For this review, take the finished solid that the model builds, in its own axes (mm). A direction names the side the tool comes from. Round coordinates to 2 decimals unless told otherwise and drop trailing zeros. Order: outer loops, then holes, each group sorted by start corner. A loop starts at its lowest first (then second) coordinate and runs counter-clockwise, first axis right, second up. Notation, with made-up numbers: (-28.5, -1.5) - (29.5, -1.5) arc R20 ccw to (29.5, 31.5) - close; hole circle Ø4 at (-9.75, 67.5). An arc over 180 degrees is marked (long way). One line per item, written item: value.
Autodesk Inventor part; units mm, degrees
ref_plane "YZ Plane" through (0, 0, 0) normal (1, 0, 0) x (0, 1, 0)
ref_plane "XZ Plane" through (0, 0, 0) normal (0, 1, 0) x (-1, 0, 0)
ref_plane "XY Plane" through (0, 0, 0) normal (0, 0, 1) x (1, 0, 0)
sketch "Sketch1" plane through (0, 0, 0) normal (0, 0, 1) x (1, 0, 0)
  line L0 (-9, 0) -> (0, 0) construction
  line L1 (-19, 0) -> (-9, 0) construction
  line L2 (-28, 0) -> (-19, 0) construction
  line L3 (0, 0) -> (-28, 0)
  line L4 (-28, 0) -> (-28, -35)
  line L5 (-28, -35) -> (0, -35)
  line L6 (0, -35) -> (0, 0)
  line L7 (-19, 0) -> (-9, 0)
  line L8 (-19, 0) -> (-19, -3)
  line L9 (-9, -3) -> (-19, -3)
  line L10 (-9, 0) -> (-9, -3)
  dimension "d0" = 35
extrude "Extrusion1" add sketch "Sketch1" along normal blind 3 contours L6 L5 L4 L3 L8 L9 L10
sketch "Sketch2" plane through (0, 0, 0) normal (0, 0, -1) x (-1, 0, 0)
  arc A0 (6.85, -9.25) -> (3.15, -9.25) centre (5, -9.25) ccw construction
  line L0 (6.85, -9.25) -> (6.85, -12.05) construction
  arc A1 (3.15, -12.05) -> (6.85, -12.05) centre (5, -12.05) ccw construction
  line L1 (3.15, -12.05) -> (3.15, -9.25) construction
  line L2 (21.15, -12.05) -> (21.15, -9.25) construction
  arc A2 (21.15, -12.05) -> (24.85, -12.05) centre (23, -12.05) ccw construction
  line L3 (24.85, -9.25) -> (24.85, -12.05) construction
  arc A3 (24.85, -9.25) -> (21.15, -9.25) centre (23, -9.25) ccw construction
  line L4 (5, -12.05) -> (5, -9.25) construction
  line L5 (5, -10.65) -> (3.15, -10.65) construction
  line L6 (23, -12.05) -> (23, -9.25) construction
  line L7 (23, -10.65) -> (21.15, -10.65) construction
  circle A4 centre (5, -10.65) radius 1.85
  circle A5 centre (23, -10.65) radius 1.85
  point P0 (0, 0)
extrude "Extrusion2" cut sketch "Sketch2" against normal blind 6.175
sketch "Sketch3" plane through (0, 0, 3) normal (0, 0, 1) x (1, 0, 0)
  line L0 (-9, -3) -> (-19, -3)
  line L1 (-28, -35) -> (0, -35)
  line L2 (-14, -3) -> (-14, -35) construction
  line L3 (-28, -35) -> (0, -35) construction
  line L4 (-14, -19) -> (0, -19) construction
  line L5 (0, -35) -> (0, 0) construction
  circle A0 centre (-14, -19) radius 2
  dimension "d5" = 4
extrude "Extrusion3" cut sketch "Sketch3" against normal blind 6.175
sketch "Sketch4" plane through (-28, -35, 0) normal (0, -1, 0) x (1, 0, 0)
  line L0 (9, 3) -> (19, 3)
  line L1 (19, 3) -> (19, 0)
  line L2 (9, 0) -> (19, 0)
  line L3 (9, 0) -> (9, 3)
  point P0 (28, 0)
extrude "Extrusion4" add sketch "Sketch4" along normal blind 3
sketch "Sketch5" plane through (0, 0, 0) normal (0, 0, -1) x (-1, 0, 0)
  arc A0 (6.85, -25.95) -> (3.15, -25.95) centre (5, -25.95) ccw construction
  line L0 (6.85, -25.95) -> (6.85, -28.75) construction
  arc A1 (3.15, -28.75) -> (6.85, -28.75) centre (5, -28.75) ccw construction
  line L1 (3.15, -28.75) -> (3.15, -25.95) construction
  arc A2 (1, -20.4) -> (0, -21.4) centre (1, -21.4) ccw construction
  line L2 (0, -21.4) -> (0, -34) construction
  line L3 (0, -34) -> (10, -34) construction
  line L4 (10, -34) -> (10, -21.4) construction
  arc A3 (10, -21.4) -> (9, -20.4) centre (9, -21.4) ccw construction
  line L5 (9, -20.4) -> (1, -20.4) construction
  arc A4 (24.85, -25.95) -> (21.15, -25.95) centre (23, -25.95) ccw construction
  line L6 (24.85, -25.95) -> (24.85, -28.75) construction
  arc A5 (21.15, -28.75) -> (24.85, -28.75) centre (23, -28.75) ccw construction
  line L7 (21.15, -28.75) -> (21.15, -25.95) construction
  arc A6 (19, -20.4) -> (18, -21.4) centre (19, -21.4) ccw construction
  line L8 (18, -21.4) -> (18, -34) construction
  line L9 (18, -34) -> (28, -34) construction
  line L10 (28, -34) -> (28, -21.4) construction
  arc A7 (28, -21.4) -> (27, -20.4) centre (27, -21.4) ccw construction
  line L11 (27, -20.4) -> (19, -20.4) construction
  line L12 (5, -28.75) -> (5, -25.95) construction
  line L13 (23, -28.75) -> (23, -25.95) construction
  circle A8 centre (5, -27.35) radius 1.85
  circle A9 centre (23, -27.35) radius 1.85
  point P0 (0, 0)
extrude "Extrusion5" cut sketch "Sketch5" against normal blind 3
properties part number "Camera mount side bars"
Item 1: Machinability: for faces 4 (the flat face through (-19, -1, 1)), 5 (the flat face through (-19, -36, 1)), 6 (the flat face through (-9, -36, 2)), which of the approach directions +Z, -Z, +X, -X, +Y, -Y give a long, thin tool a straight path to every point of the face, cutting with its end or side? Answer none if there is none.
Returned:
face 4: +Z, -Z, +Y
face 5: +Z, -Z, -X, -Y
face 6: +Z, -Z, +X, -Y
Item 2: Take a section at B-B (y = -10.65). Write out the cut boundary in (x, z).
Returned:
outline: (-28, 0) - (-24.85, 0) - (-24.85, 3) - (-28, 3) - close; (-21.15, 0) - (-6.85, 0) - (-6.85, 3) - (-21.15, 3) - close; (-3.15, 0) - (0, 0) - (0, 3) - (-3.15, 3) - close
Item 3: Wall thickness on line 1 (Y direction, x = -5, z = 1.3); line 2 (Y direction, x = -6.5, z = 2.8); line 3 (Y direction, x = -14, z = 0.7): over which ranges is each line inside the solid? List them lowest first.
Returned:
line 1: -35 to -29.2, -25.5 to -12.5, -8.8 to 0
line 2: -35 to -28.43, -26.27 to -11.73, -9.57 to 0
line 3: -38 to -21, -17 to -3
Item 4: For P1, Ø1.5, axis at y = -36, z = 1.5, coming from the -X side; P2, Ø0.9, axis at x = -14, z = 1.5, coming from the +Y side; P3, Ø0.9, axis at x = -23, z = 1.5, coming from the -Y side, all flat-tipped, find the tip position at first contact; note any pin that passes through.
Returned:
P1: x = -19
P2: y = -3
P3: y = -35
Item 5: Take a section at D-D (x = -14). Write out the cut boundary in (y, z), plus the area to 3 significant figures.
Returned:
outline: (-38, 0) - (-21, 0) - (-21, 3) - (-38, 3) - close; (-17, 0) - (-3, 0) - (-3, 3) - (-17, 3) - close
area: 93.0 mm^2
Item 6: The part is to be moulded in two halves that separate along Y. For faces 1 (the flat face through (0, -18, 1)), 2 (the cylindrical face through (-14, -17, 2)), 3 (the flat face through (-14, -38, 2)), say which applies: +Y half, -Y half, draft (parallel to the pull), parting line (faces both ways), or undercut.
Returned:
face 1: draft
face 2: undercut
face 3: -Y half
Item 7: Take a section at A-A (x = -5). Write out the cut boundary in (y, z).
Returned:
outline: (-35, 0) - (-29.2, 0) - (-29.2, 3) - (-35, 3) - close; (-25.5, 0) - (-12.5, 0) - (-12.5, 3) - (-25.5, 3) - close; (-8.8, 0) - (0, 0) - (0, 3) - (-8.8, 3) - close
Item 8: Take a section at C-C (z = 1.5). Write out the cut boundary in (x, y).
Returned:
outline: (-28, -35) - (-19, -35) - (-19, -38) - (-9, -38) - (-9, -35) - (0, -35) - (0, 0) - (-9, 0) - (-9, -3) - (-19, -3) - (-19, 0) - (-28, 0) - close; hole circle Ø3.7 at (-23, -27.35); hole circle Ø3.7 at (-23, -10.65); hole circle Ø4 at (-14, -19); hole circle Ø3.7 at (-5, -27.35); hole circle Ø3.7 at (-5, -10.65)
